Check sheet for the modelled part. Datum: model origin and axes. Units: mm. A direction names the side the tool comes from. Round coordinates to 2 decimals unless told otherwise and drop trailing zeros. Write each loop counter-clockwise with the first axis right and the second up, starting at its lowest first coordinate (ties: lowest second). Pieces come first, ordered by that corner, then holes. Notation, with made-up numbers: (-22, -28.5) - (28, -28.5) arc R13 cw to (28, -13.5) - close; hole circle Ø8 at (-25, 48.25). An arc over 180 degrees is marked (long way). Answer as a JSON object with one key per item and string values. Group by question number.
Item 1: Thickness scan on line 1 (Y direction, x = 0, z = 7.5); line 2 (Y direction, x = -15.5, z = 35); line 3 (X direction, y = -8, z = 12). Record the ranges inside material, lowest first.
Item 2: Release check for a two-part mould opening along X. For faces 4 (the flat face through (60, 0, 5)), 5 (the flat face through (0, 60, 5)), 6 (the cylindrical face through (-1.301, -46.143, 4.93)) record: pulls with the +X half, pulls with the -X half, needs draft (parallel to the pull), parting line crosses it, or undercut.
Item 3: Set-up check for faces 1 (the flat face through (10, 50, 5)), 2 (the flat face through (10, -50, 5)), 3 (the cylindrical face through (41.569, 17.235, 11.586)): record each of +Z, -Z, +X, -X, +Y, -Y from which the full face is reachable in a straight line by a thin tool's end or side.
Item 4: Sectioned sample at A-A on z = 2. Count the separate pieces of the cut face and the enclosed holes in it, plus the area to 3 significant figures.
Item 5: Gauge pin test, flat ends, axial feed: P1, Ø10, axis at y = 21.5, z = 18.5, coming from the -X side; P2, Ø5, axis at y = -49, z = 4, coming from the -X side; P3, Ø1.5, axis at x = -1, z = 33, coming from the -Y side. Record the tip position at first contact, or that the pin passes through.
Item 6: Sectioned sample at B-B on y = 52. Record the boundary of the cut face in (x, z), plus the area to 3 significant figures.
```python
from build123d import *

# Parameters (mm, degrees)
SZKIC1_R                    = 45
SZKIC1_R_2                  = 22.5
DODANIE_WYCI_GNI_CIE1_DEPTH = 41
DODANIE_WYCI_GNI_CIE2_DEPTH = 10
SZKIC3_R                    = 6
WYTNIJ_WYCI_GNI_CIE1_DEPTH  = 10
SZYK_KO_OWY1_COUNT          = 4
WYTNIJ_WYCI_GNI_CIE2_START  = -20
SZKIC5_R                    = 45
SZKIC5_R_2                  = 42.5
WYTNIJ_WYCI_GNI_CIE2_DEPTH  = 20
SZKIC6_R                    = 37.5
SZKIC6_R_2                  = 27.5
WYTNIJ_WYCI_GNI_CIE3_DEPTH  = 1
SFAZOWANIE1_SIZE            = 5


with BuildPart() as part:
    # Szkic1 → Dodanie-wyciągnięcie1 (new body)
    with BuildSketch(Plane.XY):
        Circle(SZKIC1_R)
        Circle(SZKIC1_R_2, mode=Mode.SUBTRACT)
    extrude(amount=DODANIE_WYCI_GNI_CIE1_DEPTH)

    # Szkic2 → Dodanie-wyciągnięcie2 (add)
    with BuildSketch(Plane(origin=(0, 0, 0), x_dir=(-1, 0, 0), z_dir=(0, 0, -1))):
        with BuildLine():
            Line((35, 10), (56, 10))
            ThreePointArc((56, 10), (58.828427125, 8.828427125), (60, 6))
            Line((60, 6), (60, -6))
            ThreePointArc((60, -6), (58.828427125, -8.828427125), (56, -10))
            Line((56, -10), (35, -10))
            Line((35, -10), (35, 10))
        make_face()
        with BuildLine():
            Line((-10, 35), (10, 35))
            Line((10, 35), (10, 56))
            ThreePointArc((10, 56), (8.828427125, 58.828427125), (6, 60))
            Line((6, 60), (-6, 60))
            ThreePointArc((-6, 60), (-8.828427125, 58.828427125), (-10, 56))
            Line((-10, 56), (-10, 35))
        make_face()
        with BuildLine():
            Line((10, -35), (10, -56))
            ThreePointArc((10, -56), (8.828427125, -58.828427125), (6, -60))
            Line((6, -60), (-6, -60))
            ThreePointArc((-6, -60), (-8.828427125, -58.828427125), (-10, -56))
            Line((-10, -56), (-10, -35))
            Line((-10, -35), (10, -35))
        make_face()
        with BuildLine():
            Line((-35, -10), (-56, -10))
            ThreePointArc((-56, -10), (-58.828427125, -8.828427125), (-60, -6))
            Line((-60, -6), (-60, 6))
            ThreePointArc((-60, 6), (-58.828427125, 8.828427125), (-56, 10))
            Line((-56, 10), (-35, 10))
            Line((-35, 10), (-35, -10))
        make_face()
    extrude(amount=-DODANIE_WYCI_GNI_CIE2_DEPTH)

    # Szkic3 → Wytnij-wyciągnięcie1 (cut)
    with BuildSketch(Plane(origin=(0, 0, 0), x_dir=(-1, 0, 0), z_dir=(0, 0, -1))):
        with Locations((0, 52)):
            Circle(SZKIC3_R)
    wytnij_wyci_gni_cie1 = extrude(amount=-WYTNIJ_WYCI_GNI_CIE1_DEPTH, mode=Mode.SUBTRACT)

    # Szyk kołowy1: Wytnij-wyciągnięcie1 ×4 about axis
    szyk_ko_owy1_axis = Axis((0, 0, 0), (0, 0, 1))
    for i in range(1, SZYK_KO_OWY1_COUNT):
        add(wytnij_wyci_gni_cie1.rotate(szyk_ko_owy1_axis, i * 360 / SZYK_KO_OWY1_COUNT), mode=Mode.SUBTRACT)

    # Szkic5 → Wytnij-wyciągnięcie2 (cut)
    with BuildSketch(Plane.XY.offset(41).offset(WYTNIJ_WYCI_GNI_CIE2_START)):
        with Locations(Location((0, 0, 0), (0, 0, 167.160411593))):
            Circle(SZKIC5_R)
        Circle(SZKIC5_R_2, mode=Mode.SUBTRACT)
    extrude(amount=WYTNIJ_WYCI_GNI_CIE2_DEPTH, mode=Mode.SUBTRACT)

    # Szkic6 → Wytnij-wyciągnięcie3 (cut)
    with BuildSketch(Plane.XY.offset(41)):
        Circle(SZKIC6_R)
        Circle(SZKIC6_R_2, mode=Mode.SUBTRACT)
    extrude(amount=-WYTNIJ_WYCI_GNI_CIE3_DEPTH, mode=Mode.SUBTRACT)

    # Sfazowanie1
    # the kernel refuses this chamfer: 5 mm, written as the material it adds along each edge
    with BuildSketch(Plane(origin=(0, 0, 21), x_dir=(1, 0, 0), z_dir=(0, -1, 0))) as sfazowanie1_piece_1_section:
        Polygon((42.5 + SFAZOWANIE1_SIZE, 0), (42.5, SFAZOWANIE1_SIZE), (42.5, 0), align=None)
    sfazowanie1_piece_1 = revolve(axis=Axis((0, 0, 21), (0, 0, 1)), mode=Mode.PRIVATE)
    sfazowanie1_piece_1 = sfazowanie1_piece_1 & Plane(origin=(0, 0, 24.721078182), x_dir=(1, 0, 0), z_dir=(0, 0, -1)) * Cylinder(45, 190, mode=Mode.PRIVATE)
    add(sfazowanie1_piece_1)


solid = part.part
```
Completed:
{
 "1": {"line 1": "-60 to -58, -46 to -22.5, 22.5 to 46, 58 to 60", "line 2": "-39.57 to -16.31, 16.31 to 39.57", "line 3": "-44.28 to -21.03, 21.03 to 44.28"},
 "2": {"face 4": "pulls with the +X half", "face 5": "needs draft", "face 6": "undercut"},
 "3": {"face 1": "+Z, -Z, +X, +Y", "face 2": "+Z, -Z, +X, -Y", "face 3": "+Z"},
 "4": {"separate pieces": "1", "enclosed holes": "5", "area": "5,520 mm²"},
 "5": {"P1": "x = -41.87", "P2": "x = -10", "P3": "y = -42.5"},
 "6": {"outline": "(-10, 0) - (-6, 0) - (-6, 10) - (-10, 10) - close; (6, 0) - (10, 0) - (10, 10) - (6, 10) - close", "area": "80.0 mm²"}
}
